Here's how the part is built. I have some questions about the finished solid (model axes, mm). A direction names the side the tool comes from. Round coordinates to 2 decimals unless told otherwise and drop trailing zeros. Write each loop counter-clockwise with the first axis right and the second up, starting at its lowest first coordinate (ties: lowest second). Pieces come first, ordered by that corner, then holes. Notation, with made-up numbers: (-32, 24) -> (-10, 24) arc R28 cw to (-10, 58) -> close; hole circle Ø6 at (8.25, -35). An arc over 180 degrees is marked (long way). Answer as CSV lines item,"result".
from build123d import *

# Parameters (mm, degrees)
SKETCH2_R               = 12.5
CUT_EXTRUDE1_DEPTH      = 65.031242374
BOSS_EXTRUDE1_START     = 20
SKETCH3_R               = 25
BOSS_EXTRUDE1_DEPTH     = 20
SKETCH2_2_R             = 12.5
CUT_EXTRUDE2_DEPTH      = 76.498344353
SKETCH5_R               = 20
CUT_EXTRUDE3_DEPTH      = 5
CUT_EXTRUDE3_DRAFT      = -45
SKETCH6_R               = 15
CUT_EXTRUDE4_DEPTH      = 73.284161474
CUT_EXTRUDE5_REACH      = 93.241
CUT_EXTRUDE5_END_RADIUS = 15
SKETCH10_R              = 4


with BuildPart() as part:
    # Sketch1 → Revolve1 (revolve)
    with BuildSketch(Plane.XY, mode=Mode.PRIVATE) as revolve1_sk:
        Polygon((0, 0), (0, 40), (5, 40), (10.459553514, 25), (19.540446486, 25), (25, 40), (30, 40), (30, 0), align=None)
    revolve(revolve1_sk.sketch.rotate(Axis((0, 0, 0), (1, 0, 0)), 180), axis=Axis((0, 0, 0), (1, 0, 0)))

    # Sketch2 → Cut-Extrude1 (cut, through all)
    with BuildSketch(Plane.ZY):
        with Locations(Location((0, 0, 0), (0, 0, 270))):
            Circle(SKETCH2_R)
    extrude(amount=-CUT_EXTRUDE1_DEPTH, mode=Mode.SUBTRACT)

    # Sketch3 → Boss-Extrude1 (add)
    with BuildSketch(Plane(origin=(30, 0, 0), x_dir=(0, 0, -1), z_dir=(1, 0, 0)).offset(BOSS_EXTRUDE1_START)):
        with Locations(Location((0, 0, 0), (0, 0, 270))):
            Circle(SKETCH3_R)
    extrude(amount=-BOSS_EXTRUDE1_DEPTH)

    # Sketch2<2> → Cut-Extrude2 (cut, through all)
    with BuildSketch(Plane.ZY):
        with Locations(Location((0, 0, 0), (0, 0, 270))):
            Circle(SKETCH2_2_R)
    extrude(amount=-CUT_EXTRUDE2_DEPTH, mode=Mode.SUBTRACT)


with BuildPart() as cut_extrude3_tool:
    # Sketch5 → Cut-Extrude3 (with draft: the straight prism first)
    with BuildSketch(Plane.ZY):
        Circle(SKETCH5_R)
    extrude(amount=-CUT_EXTRUDE3_DEPTH)
    # Cut-Extrude3: the draft: its side faces are tilted about the plane it starts from
    cut_extrude3_sides = [cut_extrude3_tool.faces().sort_by_distance(p)[0] for p in [
        (2.5, 0, -20),
    ]]
    draft(cut_extrude3_sides, Plane.ZY, CUT_EXTRUDE3_DRAFT)


with BuildPart() as part_1:
    add(part.part)

    # Cut-Extrude3: cut by cut_extrude3_tool
    add(cut_extrude3_tool.part, mode=Mode.SUBTRACT)

    # Sketch6 → Cut-Extrude4 (cut, through all)
    with BuildSketch(Plane.ZY.offset(-5)):
        with Locations(Location((0, 0, 0), (0, 0, 270))):
            Circle(SKETCH6_R)
    extrude(amount=-CUT_EXTRUDE4_DEPTH, mode=Mode.SUBTRACT)

    # Cut-Extrude5: up to this cylinder (the profile starts outside it)
    cut_extrude5_end = Plane(origin=(40, 0, 0), z_dir=(-1, 0, 0)) * Cylinder(CUT_EXTRUDE5_END_RADIUS, 217.482, mode=Mode.PRIVATE)
    # Sketch10 → Cut-Extrude5 (cut, up to the surface)
    with BuildSketch(Plane(origin=(0, 25, 0), x_dir=(1, 0, 0), z_dir=(0, 1, 0)), mode=Mode.PRIVATE) as cut_extrude5_sk1:
        with Locations(Location((40, 0, 0), (0, 0, 270))):
            Circle(SKETCH10_R)
    cut_extrude5_tool1 = extrude(cut_extrude5_sk1.sketch, amount=-CUT_EXTRUDE5_REACH, mode=Mode.PRIVATE) - cut_extrude5_end
    add(cut_extrude5_tool1.solids().sort_by_distance((40, 25, 0))[0], mode=Mode.SUBTRACT)


solid = part_1.part
Item 1: If we mould it in two halves opening along Z, with no side actions, what happens to faces 4 (the conical face through (4.687, -14.949, -3.32)), 5 (the flat face through (50, -11, 11)), 6 (the cylindrical face through (40.14, -23.846, -7.509)), 7 (the cylindrical face through (43.966, 19.802, -0.521))? For each: pulls with the +Z half, pulls with the -Z half, needs draft (parallel to the pull), parting line crosses it, or undercut.
Results found:
face 4,"undercut"
face 5,"needs draft"
face 6,"parting line crosses it"
face 7,"undercut"
Item 2: Suppose I cut it at A-A, the plane y = 0. List the corners of the cut face in (x, z) for me.
Results found:
outline,"(0, -40) -> (5, -40) -> (10.46, -25) -> (19.54, -25) -> (25, -40) -> (30, -40) -> (30, -25) -> (50, -25) -> (50, -15) -> (5, -15) -> (0, -20) -> close; (0, 20) -> (5, 15) -> (50, 15) -> (50, 25) -> (30, 25) -> (30, 40) -> (25, 40) -> (19.54, 25) -> (10.46, 25) -> (5, 40) -> (0, 40) -> close"
Item 3: Suppose I cut it at C-C, the plane x = 40. List the corners of the cut face in (y, z) for me.
Results found:
outline,"(14.46, -4) arc R15 cw (long way) to (14.46, 4) -> (24.68, 4) arc R25 ccw (long way) to (24.68, -4) -> close"
Item 4: I need wall thicknesses on L1, parallel to X at y = 20, z = 0; L2, parallel to Z at x = 26, y = 0; L3, parallel to Z at x = 40, y = 20. Which ranges of each line are inside material? Lowest first, please.
Results found:
L1,"x = 0 to 36, 44 to 50"
L2,"z = -40 to -15, 15 to 40"
L3,"z = -15 to -4, 4 to 15"
Item 5: For faces 1 (the cylindrical face through (27.54, 39.96, -1.76)), 2 (the conical face through (10.2, -11.9, 22.8)), 3 (the flat face through (30, -17.22, -18.34)), which set-ups out of +Z, -Z, +X, -X, +Y, -Y let a thin tool reach every point of the face, with its end or its side?
Results found:
face 1,"+X, -X"
face 2,"none"
face 3,"+X"
Item 6: Suppose I cut it at B-B, the plane z = 0. List the corners of the cut face in (x, y) for me.
Results found:
outline,"(0, -40) -> (5, -40) -> (10.46, -25) -> (19.54, -25) -> (25, -40) -> (30, -40) -> (30, -25) -> (50, -25) -> (50, -15) -> (5, -15) -> (0, -20) -> close; (0, 20) -> (5, 15) -> (36, 15) -> (36, 25) -> (30, 25) -> (30, 40) -> (25, 40) -> (19.54, 25) -> (10.46, 25) -> (5, 40) -> (0, 40) -> close; (44, 15) -> (50, 15) -> (50, 25) -> (44, 25) -> close"
Item 7: Will these pins go through, and if not, where does the flat tip stop? pin 1 (2 mm diameter, centred on x = 32, y = -27, fed in from -Z); pin 2 (1.5 mm diameter, centred on x = 5.5, z = -15, fed in from -Y); pin 3 (2 mm diameter, centred on y = -15.5, z = -6.5, fed in from -X); pin 4 (9 mm diameter, centred on x = 40, z = 0, fed in from +Y).
Results found:
pin 1,"passes through"
pin 2,"stops at y = -37.3"
pin 3,"stops at x = 2.19"
pin 4,"stops at y = 25"
